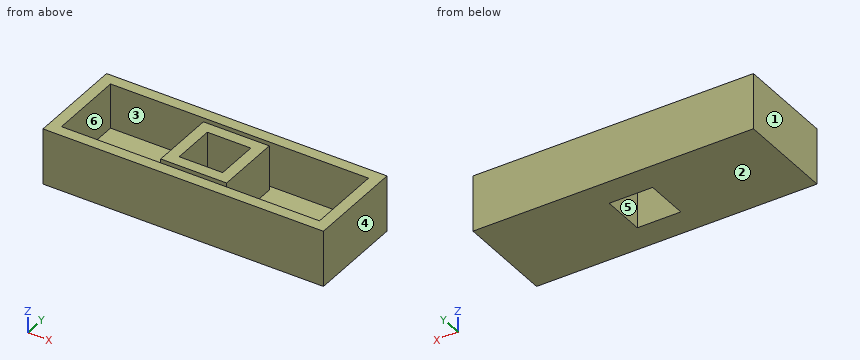
```python
from build123d import *

# Parameters (mm, degrees)
SKETCH1_W           = 20
SKETCH1_H           = 7
SKETCH1_W_2         = 3.1
SKETCH1_H_2         = 3.1
BOSS_EXTRUDE1_DEPTH = 4
SHELL1_T            = -0.8


with BuildPart() as part:
    # Sketch1 → Boss-Extrude1 (new body)
    with BuildSketch(Plane.XY):
        with Locations((1.55, 1.55)):
            Rectangle(SKETCH1_W, SKETCH1_H)
        with Locations((1.55, 1.55)):
            Rectangle(SKETCH1_W_2, SKETCH1_H_2, mode=Mode.SUBTRACT)
    extrude(amount=BOSS_EXTRUDE1_DEPTH)

    # Shell1
    shell1_openings = [part.faces().sort_by_distance(p)[0] for p in [
        (1.55, -1.738103799, 4),
    ]]
    offset(amount=SHELL1_T, openings=shell1_openings, kind=Kind.INTERSECTION)


solid = part.part
```
For this review, take the finished solid that the model builds, in its own axes (mm). Face numbers are marked on the shaded views. A direction names the side the tool comes from. Round coordinates to 2 decimals unless told otherwise and drop trailing zeros. Write each loop counter-clockwise with the first axis right and the second up, starting at its lowest first coordinate (ties: lowest second). Pieces come first, ordered by that corner, then holes. Notation, with made-up numbers: (49, -18.5) -> (55, -18.5) arc R15 ccw to (55, 5.5) -> close; hole circle Ø5 at (16.25, -14.5). An arc over 180 degrees is marked (long way). One line per question, with ' | ' between items. Start each with the question number.
(1) Add section C-C, the plane y = 1.25. Write out the cut boundary in (x, z), plus the area to 3 significant figures.
(2) Tool access review of the marked faces 4, 5 and 6: name each direction out of +Z, -Z, +X, -X, +Y, -Y from which nothing blocks a thin tool from reaching the whole face with its end or side.
(3) Mouldability with a two-part tool opening along X and no side actions: class the marked faces 1, 2 and 3 as released by +X, released by -X, zero draft, split by the parting line, or undercut.
(4) Add section A-A, the plane x = 1.5. Write out the cut boundary in (y, z).
(5) Add section D-D, the plane z = 0.3. Write out the cut boundary in (x, y), plus the area to 3 significant figures.
(6) Insertion check: P1, Ø2.5, axis at x = -3, y = 1, coming from the +Z side. The pin has a flat end and moves straight along its axis. Give the tip position at first contact, or say it passes through.
(7) For line 1 along X through (y, z) = (0.25, 1.45); line 2 along X through (y, z) = (3.25, 2.1); line 3 along Y through (x, z) = (1.75, 1), list the stretches that pass through material, from the lowest coordinate up. Write a range as from..to.
(8) Add section B-B, the plane z = 3.7. Write out the cut boundary in (x, y).
Answer list:
1) outline: (-8.45, 0) -> (0, 0) -> (0, 4) -> (-0.8, 4) -> (-0.8, 0.8) -> (-7.65, 0.8) -> (-7.65, 4) -> (-8.45, 4) -> close; (3.1, 0) -> (11.55, 0) -> (11.55, 4) -> (10.75, 4) -> (10.75, 0.8) -> (3.9, 0.8) -> (3.9, 4) -> (3.1, 4) -> close | area: 23.8 mm²
2) face 4: +Z, -Z, +X, +Y, -Y | face 5: +Z, -Z | face 6: +Z
3) face 1: released by -X | face 2: zero draft | face 3: undercut
4) outline: (-1.95, 0) -> (0, 0) -> (0, 4) -> (-0.8, 4) -> (-0.8, 0.8) -> (-1.15, 0.8) -> (-1.15, 4) -> (-1.95, 4) -> close; (3.1, 0) -> (5.05, 0) -> (5.05, 4) -> (4.25, 4) -> (4.25, 0.8) -> (3.9, 0.8) -> (3.9, 4) -> (3.1, 4) -> close
5) outline: (-8.45, -1.95) -> (11.55, -1.95) -> (11.55, 5.05) -> (-8.45, 5.05) -> close; hole (0, 0) -> (3.1, 0) -> (3.1, 3.1) -> (0, 3.1) -> close | area: 130 mm²
6) P1: z = 0.8
7) line 1: -8.45..-7.65, -0.8..0, 3.1..3.9, 10.75..11.55 | line 2: -8.45..-7.65, -0.8..3.9, 10.75..11.55 | line 3: -1.95..-1.15, -0.8..0, 3.1..3.9, 4.25..5.05
8) outline: (-8.45, -1.95) -> (11.55, -1.95) -> (11.55, 5.05) -> (-8.45, 5.05) -> close; (-0.8, -0.8) -> (3.9, -0.8) -> (3.9, 3.9) -> (-0.8, 3.9) -> close; hole (-7.65, -1.15) -> (10.75, -1.15) -> (10.75, 4.25) -> (-7.65, 4.25) -> close; hole (0, 0) -> (3.1, 0) -> (3.1, 3.1) -> (0, 3.1) -> close
